```python
from build123d import *

# Parameters (mm, degrees)
SKETCH1_R           = 2.625
BOSS_EXTRUDE1_DEPTH = 3.175


with BuildPart() as part:
    # Sketch1 → Boss-Extrude1 (new body)
    with BuildSketch(Plane.XY):
        with BuildLine():
            Line((4.813695848, 148.856298887), (4.813695848, 136.524994751))
            ThreePointArc((4.813695848, 136.524994751), (5.557644624, 134.728943527), (7.353695848, 133.984994751))
            Line((7.353695848, 133.984994751), (8.813799985, 133.984994751))
            ThreePointArc((8.813799985, 133.984994751), (10.609851209, 133.241045975), (11.353799985, 131.444994751))
            Line((11.353799985, 131.444994751), (11.353799985, 112.775997772))
            ThreePointArc((11.353799985, 112.775997772), (10.609851209, 110.979946548), (8.813799985, 110.235997772))
            Line((8.813799985, 110.235997772), (4.813695848, 110.235997772))
            ThreePointArc((4.813695848, 110.235997772), (-1.536304152, 103.885997772), (4.813695848, 97.535997772))
            Line((4.813695848, 97.535997772), (8.813799985, 97.535997772))
            ThreePointArc((8.813799985, 97.535997772), (10.609851209, 96.792048996), (11.353799985, 94.995997772))
            Line((11.353799985, 94.995997772), (11.353799985, 76.327000793))
            ThreePointArc((11.353799985, 76.327000793), (10.609851209, 74.530949569), (8.813799985, 73.787000793))
            Line((8.813799985, 73.787000793), (7.353695848, 73.787000793))
            ThreePointArc((7.353695848, 73.787000793), (5.557644624, 73.043052018), (4.813695848, 71.247000793))
            Line((4.813695848, 71.247000793), (4.813695848, 58.915696657))
            ThreePointArc((4.813695848, 58.915696657), (6.673567788, 54.425568596), (11.163695848, 52.565696657))
            Line((11.163695848, 52.565696657), (23.494999985, 52.565696657))
            ThreePointArc((23.494999985, 52.565696657), (25.291051209, 53.309645433), (26.034999985, 55.105696657))
            Line((26.034999985, 55.105696657), (26.034999985, 56.565800793))
            ThreePointArc((26.034999985, 56.565800793), (26.778948761, 58.361852018), (28.574999985, 59.105800793))
            Line((28.574999985, 59.105800793), (43.179998741, 59.105800793))
            ThreePointArc((43.179998741, 59.105800793), (44.976049965, 58.361852018), (45.719998741, 56.565800793))
            Line((45.719998741, 56.565800793), (45.719998741, 52.755800793))
            ThreePointArc((45.719998741, 52.755800793), (52.069998741, 46.405800793), (58.419998741, 52.755800793))
            Line((58.419998741, 52.755800793), (58.419998741, 56.565800793))
            ThreePointArc((58.419998741, 56.565800793), (59.163947517, 58.361852018), (60.959998741, 59.105800793))
            Line((60.959998741, 59.105800793), (75.564997498, 59.105800793))
            ThreePointArc((75.564997498, 59.105800793), (77.361048722, 58.361852018), (78.104997498, 56.565800793))
            Line((78.104997498, 56.565800793), (78.104997498, 55.105696657))
            ThreePointArc((78.104997498, 55.105696657), (78.848946273, 53.309645433), (80.644997498, 52.565696657))
            Line((80.644997498, 52.565696657), (92.976301634, 52.565696657))
            ThreePointArc((92.976301634, 52.565696657), (97.466429695, 54.425568596), (99.326301634, 58.915696657))
            Line((99.326301634, 58.915696657), (99.326301634, 71.247000793))
            ThreePointArc((99.326301634, 71.247000793), (98.582352858, 73.043052018), (96.786301634, 73.787000793))
            Line((96.786301634, 73.787000793), (95.326197498, 73.787000793))
            ThreePointArc((95.326197498, 73.787000793), (93.530146273, 74.530949569), (92.786197498, 76.327000793))
            Line((92.786197498, 76.327000793), (92.786197498, 94.995997772))
            ThreePointArc((92.786197498, 94.995997772), (93.530146273, 96.792048996), (95.326197498, 97.535997772))
            Line((95.326197498, 97.535997772), (99.326301634, 97.535997772))
            ThreePointArc((99.326301634, 97.535997772), (105.676301634, 103.885997772), (99.326301634, 110.235997772))
            Line((99.326301634, 110.235997772), (95.326197498, 110.235997772))
            ThreePointArc((95.326197498, 110.235997772), (93.530146273, 110.979946548), (92.786197498, 112.775997772))
            Line((92.786197498, 112.775997772), (92.786197498, 131.444994751))
            ThreePointArc((92.786197498, 131.444994751), (93.530146273, 133.241045975), (95.326197498, 133.984994751))
            Line((95.326197498, 133.984994751), (96.786301634, 133.984994751))
            ThreePointArc((96.786301634, 133.984994751), (98.582352858, 134.728943527), (99.326301634, 136.524994751))
            Line((99.326301634, 136.524994751), (99.326301634, 148.856298887))
            ThreePointArc((99.326301634, 148.856298887), (97.466429695, 153.346426948), (92.976301634, 155.206298887))
            Line((92.976301634, 155.206298887), (80.644997498, 155.206298887))
            ThreePointArc((80.644997498, 155.206298887), (78.848946273, 154.462350112), (78.104997498, 152.666298887))
            Line((78.104997498, 152.666298887), (78.104997498, 151.206194751))
            ThreePointArc((78.104997498, 151.206194751), (77.361048722, 149.410143527), (75.564997498, 148.666194751))
            Line((75.564997498, 148.666194751), (60.959998741, 148.666194751))
            ThreePointArc((60.959998741, 148.666194751), (59.163947517, 149.410143527), (58.419998741, 151.206194751))
            Line((58.419998741, 151.206194751), (58.419998741, 155.016194751))
            ThreePointArc((58.419998741, 155.016194751), (52.069998741, 161.366194751), (45.719998741, 155.016194751))
            Line((45.719998741, 155.016194751), (45.719998741, 151.206194751))
            ThreePointArc((45.719998741, 151.206194751), (44.976049965, 149.410143527), (43.179998741, 148.666194751))
            Line((43.179998741, 148.666194751), (28.574999985, 148.666194751))
            ThreePointArc((28.574999985, 148.666194751), (26.778948761, 149.410143527), (26.034999985, 151.206194751))
            Line((26.034999985, 151.206194751), (26.034999985, 152.666298887))
            ThreePointArc((26.034999985, 152.666298887), (25.291051209, 154.462350112), (23.494999985, 155.206298887))
            Line((23.494999985, 155.206298887), (11.163695848, 155.206298887))
            ThreePointArc((11.163695848, 155.206298887), (6.673567788, 153.346426948), (4.813695848, 148.856298887))
        make_face()
        with Locations((11.163695848, 148.856298887)):
            Circle(SKETCH1_R, mode=Mode.SUBTRACT)
        with Locations((92.976301634, 148.856298887)):
            Circle(SKETCH1_R, mode=Mode.SUBTRACT)
        with Locations((52.069998741, 155.016194751)):
            Circle(SKETCH1_R, mode=Mode.SUBTRACT)
        with Locations((99.326301634, 103.885997772)):
            Circle(SKETCH1_R, mode=Mode.SUBTRACT)
        with Locations((92.976301634, 58.915696657)):
            Circle(SKETCH1_R, mode=Mode.SUBTRACT)
        with Locations((52.069998741, 52.755800793)):
            Circle(SKETCH1_R, mode=Mode.SUBTRACT)
        with Locations((11.163695848, 58.915696657)):
            Circle(SKETCH1_R, mode=Mode.SUBTRACT)
        with Locations((4.813695848, 103.885997772)):
            Circle(SKETCH1_R, mode=Mode.SUBTRACT)
    extrude(amount=BOSS_EXTRUDE1_DEPTH)


solid = part.part
```
CAD build for the part. Positions are in the model's coordinates, mm. A direction names the side the tool comes from. Coordinates: 2 decimals unless noted, no trailing zeros. Write each loop counter-clockwise with the first axis right and the second up, starting at its lowest first coordinate (ties: lowest second). Pieces come first, ordered by that corner, then holes.
(1) Two-plate mould, pull along Y, no slides. Class faces 4 (the face through (93.51, 96.77, 1.57)), 5 (the face through (36, 148.666, 2)), 6 (the face through (12.57, 61.13, 1.57)), 7 (the face through (59.14, 58.34, 1.57)): +Y half, -Y half, draft (parallel to the pull), parting line (faces both ways), or undercut.
(2) Cut at C-C, the plane x = 86. List the corners of the cut face in (y, z) (3 decimals), and give its area (3 significant figures).
(3) Drill centre lines: probe 1 along X at (y, z) = (148.5, 0.9); probe 2 along X at (y, z) = (54.5, 1.2); probe 3 along Y at (x, z) = (73.5, 0.4). Where is each one in solid material? Low to high.
(4) 3-axis set-ups, long thin cutter, end or side, ignore diameter. For faces 1 (the face through (45.72, 153, 2)), 2 (the face through (77.34, 58.38, 1.57)), 3 (the face through (92.786, 86, 2)): which of +Z, -Z, +X, -X, +Y, -Y reach the whole face in a straight line?
(5) Flat gauge pins, fed straight in: pin 1 (1 mm diameter, centred on y = 55, z = 1, fed in from +X); pin 2 (1.6 mm diameter, centred on y = 63, z = 1.5, fed in from +X); pin 3 (1.6 mm diameter, centred on x = 97.5, z = 1.5, fed in from +Y); pin 4 (4.5 mm diameter, centred on x = 11.16, y = 58.92, fed in from +Z). Where does each tip first touch, or does it go through?
(6) Cut at B-B, the plane y = 120. List the corners of the cut face in (x, z) (3 decimals).
(7) Cut at D-D, the plane z = 2.1. Count the separate pieces of the cut face and the enclosed holes in it, and give its area (3 significant figures).
(8) Cut at A-A, the plane x = 52. List the corners of the cut face in (y, z) (3 decimals), and give its area (3 significant figures).
Geometry says:
1. face 4: undercut
1. face 5: +Y half
1. face 6: undercut
1. face 7: -Y half
2. outline: (52.566, 0) - (155.206, 0) - (155.206, 3.175) - (52.566, 3.175) - close
2. area: 326 mm2
3. probe 1: x = 4.81 to 8.56, 13.76 to 90.38, 95.58 to 99.33
3. probe 2: x = 6.6 to 25.96, 45.72 to 50.11, 54.03 to 58.42, 78.18 to 97.54
3. probe 3: y = 59.11 to 148.67
4. face 1: +Z, -Z, +Y
4. face 2: +Z, -Z, -Y
4. face 3: +Z, -Z, +X
5. pin 1: stops at x = 98.33
5. pin 2: stops at x = 99.33
5. pin 3: stops at y = 154
5. pin 4: passes through
6. outline: (11.354, 0) - (92.786, 0) - (92.786, 3.175) - (11.354, 3.175) - close
7. separate pieces: 1
7. enclosed holes: 8
7. area: 8,620 mm2
8. outline: (46.406, 0) - (50.132, 0) - (50.132, 3.175) - (46.406, 3.175) - close; (55.38, 0) - (152.392, 0) - (152.392, 3.175) - (55.38, 3.175) - close; (157.64, 0) - (161.366, 0) - (161.366, 3.175) - (157.64, 3.175) - close
8. area: 332 mm2
